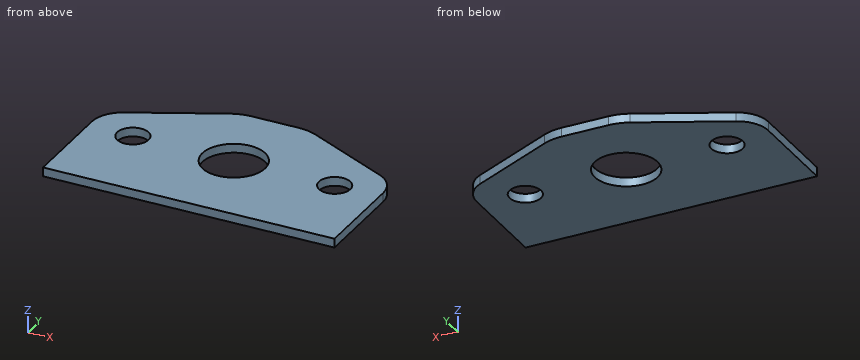
from build123d import *

# Parameters (mm, degrees)
SKETCH1_R           = 7
SKETCH1_R_2         = 3.5
BOSS_EXTRUDE1_DEPTH = 2


with BuildPart() as part:
    # Sketch1 → Boss-Extrude1 (new body)
    with BuildSketch(Plane.XY):
        with BuildLine():
            Line((-32.5, -12.7), (32.5, -12.7))
            Line((32.5, -12.7), (32.5, 8.595362211))
            ThreePointArc((32.5, 8.595362211), (31.424686587, 12.323376272), (28.529117473, 14.906023613))
            Line((28.529117473, 14.906023613), (9.551602969, 24.015230575))
            ThreePointArc((9.551602969, 24.015230575), (7.443266635, 24.750700122), (5.224292294, 25))
            Line((5.224292294, 25), (-5.224292294, 25))
            ThreePointArc((-5.224292294, 25), (-7.443266635, 24.750700122), (-9.551602969, 24.015230575))
            Line((-9.551602969, 24.015230575), (-28.529117473, 14.906023613))
            ThreePointArc((-28.529117473, 14.906023613), (-31.424686587, 12.323376272), (-32.5, 8.595362211))
            Line((-32.5, 8.595362211), (-32.5, -12.7))
        make_face()
        with Locations((0, 7)):
            Circle(SKETCH1_R, mode=Mode.SUBTRACT)
        with Locations((-22.5, 7)):
            Circle(SKETCH1_R_2, mode=Mode.SUBTRACT)
        with Locations((22.5, 7)):
            Circle(SKETCH1_R_2, mode=Mode.SUBTRACT)
    extrude(amount=BOSS_EXTRUDE1_DEPTH)


solid = part.part
Geometry check sheet. Reference: the model listing, model coordinates, mm. Give positions to 0.01 mm unless a question says otherwise; leave off trailing zeros. Loops run counter-clockwise (first coordinate to the right, second up) from the corner with the lowest first, then second, coordinate; pieces in that order, holes last. Notation, with made-up numbers: (88.25, -36.75) -> (95.25, -36.75) arc R26 cw to (95.25, -4.75) -> close; hole circle Ø9 at (-13, 75.25). An arc over 180 degrees is marked (long way). Answer in a Markdown table with one row per item. Add a question column.
1) Cross-section at D-D on x = 0. Record the boundary of the cut face in (y, z), and give its area (3 significant figures).
2) Cross-section at A-A on x = 22.5. Record the boundary of the cut face in (y, z).
3) Material ranges on probe 1 along Y at (x, z) = (0, 1.2); probe 2 along Y at (x, z) = (-2, 0.95); probe 3 along X at (y, z) = (1, 0.25), recorded low to high. Write a range as from..to.
4) Cross-section at B-B on z = 0.9. Record the boundary of the cut face in (x, y).
5) Cross-section at C-C on y = 7. Record the boundary of the cut face in (x, z), and give its area (3 significant figures).
Outcome:
| question | item | result |
|---|---|---|
| 1 | outline | (-12.7, 0) -> (0, 0) -> (0, 2) -> (-12.7, 2) -> close; (14, 0) -> (25, 0) -> (25, 2) -> (14, 2) -> close |
| 1 | area | 47.4 mm^2 |
| 2 | outline | (-12.7, 0) -> (3.5, 0) -> (3.5, 2) -> (-12.7, 2) -> close; (10.5, 0) -> (17.8, 0) -> (17.8, 2) -> (10.5, 2) -> close |
| 3 | probe 1 | y = -12.7..0, 14..25 |
| 3 | probe 2 | y = -12.7..0.29, 13.71..25 |
| 3 | probe 3 | x = -32.5..-3.61, 3.61..32.5 |
| 4 | outline | (-32.5, -12.7) -> (32.5, -12.7) -> (32.5, 8.6) arc R7 ccw to (28.53, 14.91) -> (9.55, 24.02) arc R10 ccw to (5.22, 25) -> (-5.22, 25) arc R10 ccw to (-9.55, 24.02) -> (-28.53, 14.91) arc R7 ccw to (-32.5, 8.6) -> close; hole circle Ø7 at (-22.5, 7); hole circle Ø14 at (0, 7); hole circle Ø7 at (22.5, 7) |
| 5 | outline | (-32.5, 0) -> (-26, 0) -> (-26, 2) -> (-32.5, 2) -> close; (-19, 0) -> (-7, 0) -> (-7, 2) -> (-19, 2) -> close; (7, 0) -> (19, 0) -> (19, 2) -> (7, 2) -> close; (26, 0) -> (32.5, 0) -> (32.5, 2) -> (26, 2) -> close |
| 5 | area | 74.0 mm^2 |
